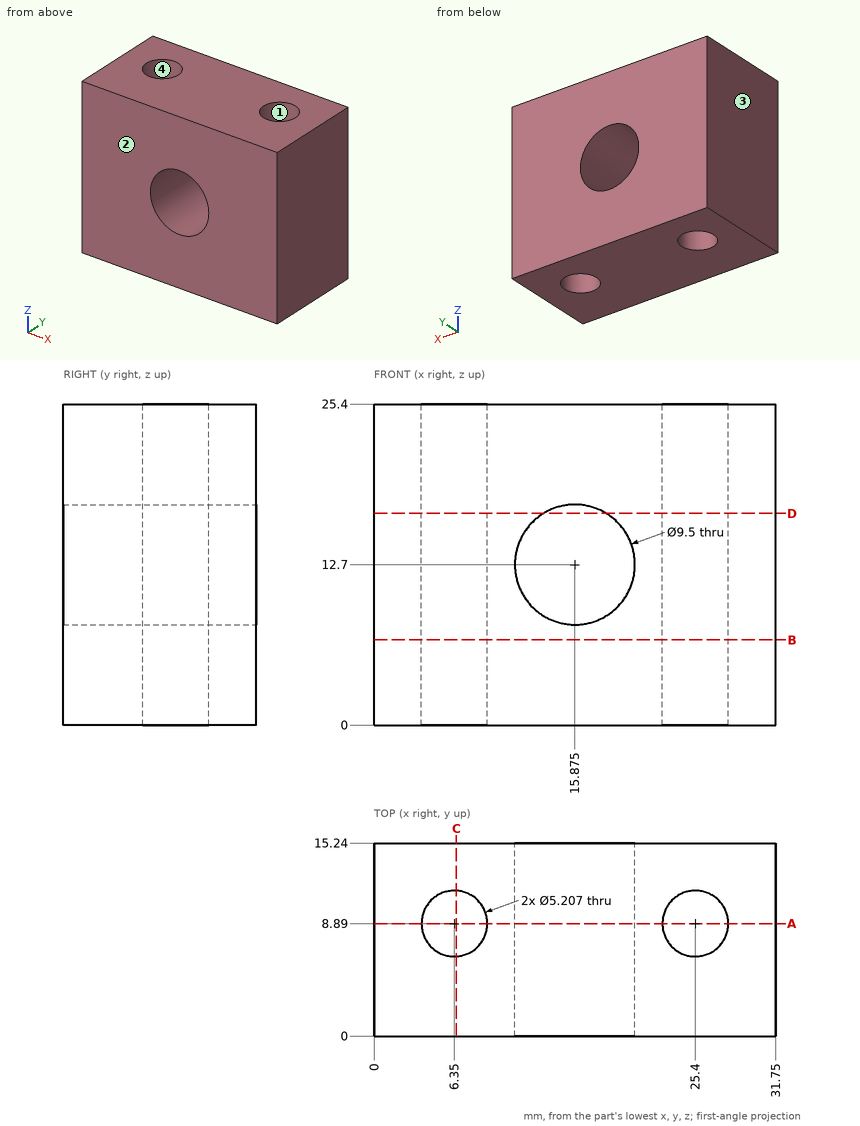
Print and shaded views of the part. All mm, measured from the part's lowest x, y and z. Round coordinates to 2 decimals unless told otherwise and drop trailing zeros. Write each loop counter-clockwise with the first axis right and the second up, starting at its lowest first coordinate (ties: lowest second). Pieces come first, ordered by that corner, then holes.
(1) Mould opens along Y. For the marked faces 1, 2, 3 and 4 say: pulls with the +Y half, pulls with the -Y half, needs draft (parallel to the pull), parting line crosses it, or undercut.
(2) Probe line 1 along X through (y, z) = (9.75, 4.75); line 2 along Y through (x, z) = (6.35, 16.25); line 3 along X through (y, z) = (7.25, 20.5). List the from-to ranges inside material, lowest first.
(3) Slice it at C-C, the plane x = 6.5. Write the cut outline in (y, z).
(4) Slice it at A-A, the plane y = 8.89. Count the separate pieces of the cut face and the enclosed holes in it, and give its area (3 significant figures).
(5) Slice it at B-B, the plane z = 6.75. Write the cut outline in (x, y), and give its area (3 significant figures).
(6) Slice it at D-D, the plane z = 16.75. Write the cut outline in (x, y), and give its area (3 significant figures).
From the geometry:
1. face 1: undercut
1. face 2: pulls with the -Y half
1. face 3: needs draft
1. face 4: undercut
2. line 1: x = 0 to 3.89, 8.81 to 22.94, 27.86 to 31.75
2. line 2: y = 0 to 6.29, 11.49 to 15.24
2. line 3: x = 0 to 4.33, 8.37 to 23.38, 27.42 to 31.75
3. outline: (0, 0) - (6.29, 0) - (6.29, 25.4) - (0, 25.4) - close; (11.49, 0) - (15.24, 0) - (15.24, 25.4) - (11.49, 25.4) - close
4. separate pieces: 3
4. enclosed holes: 1
4. area: 471 mm2
5. outline: (0, 0) - (31.75, 0) - (31.75, 15.24) - (0, 15.24) - close; hole circle Ø5.21 at (6.35, 8.89); hole circle Ø5.21 at (25.4, 8.89)
5. area: 441 mm2
6. outline: (0, 0) - (13.39, 0) - (13.39, 15.24) - (0, 15.24) - close; (18.36, 0) - (31.75, 0) - (31.75, 15.24) - (18.36, 15.24) - close; hole circle Ø5.21 at (6.35, 8.89); hole circle Ø5.21 at (25.4, 8.89)
6. area: 366 mm2
